from build123d import *

# Parameters (mm, degrees)
CROQUIS1_W              = 7
CROQUIS1_H              = 3
CROQUIS1_W_2            = 40
SALIENTE_EXTRUIR2_DEPTH = 3


with BuildPart() as part:
    # Croquis1 → Saliente-Extruir2 (new body)
    # profile 1 of 2: a face of its own
    with BuildSketch(Plane.XY):
        with BuildLine():
            Line((-6.216662119, 22.772706787), (-4.044005239, 19.70673965))
            ThreePointArc((-4.044005239, 19.70673965), (0.846790636, 15.302410265), (7.152221482, 13.415735026))
            ThreePointArc((7.152221482, 13.415735026), (31.588023052, 12.711932525), (56, 14))
            ThreePointArc((56, 14), (59.681690996, 14.144560896), (63.331119209, 13.637194987))
            Line((63.331119209, 13.637194987), (63.331119209, -13.72746384))
            ThreePointArc((63.331119209, -13.72746384), (59.669008788, -13.956513649), (56, -14))
            ThreePointArc((56, -14), (28, -10.687617167), (0, -14))
            ThreePointArc((0, -14), (-8.837271963, -10.858297484), (-13.708246846, -2.843232035))
            ThreePointArc((-13.708246846, -2.843232035), (-14.641013119, 0.09458105), (-16.154579725, 2.779709497))
            ThreePointArc((-16.154579725, 2.779709497), (-19.611540214, 8.64494659), (-22.043834508, 15.003840083))
            ThreePointArc((-22.043834508, 15.003840083), (-25.456865091, 18.879465716), (-29.94492332, 21.43418393))
            ThreePointArc((-29.94492332, 21.43418393), (-30.498768872, 21.56832041), (-31.068602309, 21.573549568))
            ThreePointArc((-31.068602309, 21.573549568), (-37.926515157, 21.320049962), (-44.755343643, 22.000000093))
            ThreePointArc((-44.755343643, 22.000000093), (-46.844869797, 22.679955064), (-48.825598798, 23.631359783))
            ThreePointArc((-48.825598798, 23.631359783), (-48.970768016, 23.707234664), (-49.120594345, 23.773440183))
            ThreePointArc((-49.120594345, 23.773440183), (-50.676363257, 25.877313669), (-49.50357007, 28.216385428))
            Line((-49.50357007, 28.216385428), (-45.399966171, 30.762281564))
            ThreePointArc((-45.399966171, 30.762281564), (-37.171530842, 35.026305913), (-27.955174947, 35.999874419))
            ThreePointArc((-27.955174947, 35.999874419), (-15.716017532, 31.637687979), (-6.216662119, 22.772706787))
        make_face()
        with Locations((-34, 26.5)):
            Rectangle(CROQUIS1_W, CROQUIS1_H, mode=Mode.SUBTRACT)
        Rectangle(CROQUIS1_W, CROQUIS1_H, mode=Mode.SUBTRACT)
        with Locations((56, 0)):
            Rectangle(CROQUIS1_W, CROQUIS1_H, mode=Mode.SUBTRACT)
        with Locations((28, 5.383929272)):
            Rectangle(CROQUIS1_W_2, CROQUIS1_H, mode=Mode.SUBTRACT)
    # profile 2 of 2: a face of its own
    with BuildSketch(Plane.XY):
        with BuildLine():
            Line((-30.68397036, 35.522018262), (-28.310242026, 42.522018262))
            ThreePointArc((-28.310242026, 42.522018262), (-27.333748746, 43.003952774), (-26.851814233, 42.027459494))
            Line((-26.851814233, 42.027459494), (-29.225542567, 35.027459494))
            ThreePointArc((-29.225542567, 35.027459494), (-30.202035847, 34.545524982), (-30.68397036, 35.522018262))
        make_face()
    extrude(amount=SALIENTE_EXTRUIR2_DEPTH)


solid = part.part
For this review, take the finished solid that the model builds, in its own axes (mm). A direction names the side the tool comes from. Round coordinates to 2 decimals unless told otherwise and drop trailing zeros. Loops run counter-clockwise (first coordinate to the right, second up) from the corner with the lowest first, then second, coordinate; pieces in that order, holes last. Notation, with made-up numbers: (78.25, 58.5) - (132.25, 58.5) arc R15 ccw to (132.25, 72.5) - close; hole circle Ø6 at (17, -7.75). An arc over 180 degrees is marked (long way). Answer as CSV lines item,"result".
(1) Consider section C-C on z = 1.95. Give the number of separate pieces and of enclosed holes in the cut face, then the cut area to 3 significant figures.
Checked values:
separate pieces,"1"
enclosed holes,"4"
area,"2,490 mm2"
(2) Mouldability with a two-part tool opening along Y and no side actions: class faces 3 (the face through (-47.48, 29.47, 1.48)), 4 (the face through (8, 5, 1)), 5 (the face through (20, 2, 0)) as +Y half, -Y half, draft (parallel to the pull), parting line (faces both ways), or undercut.
Checked values:
face 3,"+Y half"
face 4,"undercut"
face 5,"draft"
(3) Consider section D-D on x = 46. Give the boundary of the cut face in (y, z), then the cut area to 3 significant figures.
Checked values:
outline,"(-12.05, 0) - (3.88, 0) - (3.88, 3) - (-12.05, 3) - close; (6.88, 0) - (13.23, 0) - (13.23, 3) - (6.88, 3) - close"
area,"66.8 mm2"
(4) Tool access review of faces 1 (the face through (-29.42, 39.25, 1.48)), 2 (the face through (0, 1.5, 1)): name each direction out of +Z, -Z, +X, -X, +Y, -Y from which nothing blocks a thin tool from reaching the whole face with its end or side.
Checked values:
face 1,"+Z, -Z, -X, +Y"
face 2,"+Z, -Z"
(5) Insertion check: P1, Ø1.5, axis at x = 0.5, z = 2, coming from the -Y side; P2, Ø1, axis at x = -9.5, z = 1, coming from the +Y side; P3, Ø1.5, axis at x = -1, z = 1, coming from the +Y side. Each pin has a flat end and moves straight along its axis. Give the tip position at first contact, or say it passes through.
Checked values:
P1,"stops at y = -14"
P2,"stops at y = 27.2"
P3,"stops at y = 17.15"
(6) Consider section B-B on y = 0. Give the boundary of the cut face in (x, z).
Checked values:
outline,"(-14.6, 0) - (-3.5, 0) - (-3.5, 3) - (-14.6, 3) - close; (3.5, 0) - (52.5, 0) - (52.5, 3) - (3.5, 3) - close; (59.5, 0) - (63.33, 0) - (63.33, 3) - (59.5, 3) - close"
(7) Consider section A-A on x = 18. Give the boundary of the cut face in (y, z) (3 decimals).
Checked values:
outline,"(-11.105, 0) - (3.884, 0) - (3.884, 3) - (-11.105, 3) - close; (6.884, 0) - (12.857, 0) - (12.857, 3) - (6.884, 3) - close"
(8) Wall thickness on line 1 (X direction, y = 1, z = 0.6); line 2 (Y direction, x = -31, z = 2.15); line 3 (X direction, y = 0.5, z = 1.15): over which ranges is each line inside the solid? List them lowest first.
Checked values:
line 1,"x = -15.07 to -3.5, 3.5 to 52.5, 59.5 to 63.33"
line 2,"y = 21.58 to 25, 28 to 36.06"
line 3,"x = -14.82 to -3.5, 3.5 to 52.5, 59.5 to 63.33"
